from build123d import *

# Parameters (mm, degrees)
BOSS_EXTRUDE2_DEPTH = 8


with BuildPart() as part:
    # Sketch1 → Boss-Extrude2 (new body)
    with BuildSketch(Plane.XY):
        Polygon((0, 0), (-20, 0), (-20, 6), (-24, 6), (-24, 0), (-34.5, 0), (-34.5, 6), (-38.5, 6), (-38.5, -4), (0, -4), align=None)
    extrude(amount=BOSS_EXTRUDE2_DEPTH)

    # Mirror1: part across plane


with BuildPart() as part_1:
    add(part.part)
    add(part.part.mirror(Plane(origin=(0, 0, 0), x_dir=(0, 0, 1), z_dir=(1, 0, 0))))


solid = part_1.part
Could you check a few things on this model? Use its own coordinates, in mm. A direction names the side the tool comes from. Give positions to 0.01 mm unless a question says otherwise; leave off trailing zeros. Order: outer loops, then holes, each group sorted by start corner. A loop starts at its lowest first (then second) coordinate and runs counter-clockwise, first axis right, second up. Notation, with made-up numbers: (74.5, 14.5) -> (133.5, 14.5) arc R24 cw to (133.5, 37.5) -> close; hole circle Ø6 at (76.25, 36.5). An arc over 180 degrees is marked (long way). Answer in a Markdown table with one row per item. Add a question column.
Item 1: Imagine slicing it at A-A (y = 1). List the corners of the cut face in (x, z) for me.
Item 2: We'd pull the mould along X, two halves only. Please class faces 1 (the flat face through (38.5, 1, 4)), 2 (the flat face through (-24, 3, 4)), 3 (the flat face through (36, 6, 4)): pulls with the +X half, pulls with the -X half, needs draft (parallel to the pull), parting line crosses it, or undercut.
Item 3: For faces 4 (the flat face through (20, 3, 4)), 5 (the flat face through (1, -1, 0)), which set-ups out of +Z, -Z, +X, -X, +Y, -Y let a thin tool reach every point of the face, with its end or its side?
Item 4: Please list where these lines run through material, in increasing order: probe 1 along X at (y, z) = (3.25, 2.5); probe 2 along Y at (x, z) = (-19, 0.5).
Item 5: I'm going to push flat-ended pins straight in: P1, Ø3, axis at x = -30, z = 3, coming from the +Y side; P2, Ø2, axis at x = -30, y = 2, coming from the +Z side; P3, Ø4, axis at x = -25.5, y = 1, coming from the -Z side. Where does each tip first touch, or does it pass through?
Item 6: Imagine slicing it at B-B (z = 2.75). List the corners of the cut face in (x, y) for me.
Item 7: Imagine slicing it at C-C (x = -10). List the corners of the cut face in (y, z) for me.
Result:
| question | item | result |
|---|---|---|
| 1 | outline | (-38.5, 0) -> (-34.5, 0) -> (-34.5, 8) -> (-38.5, 8) -> close; (-24, 0) -> (-20, 0) -> (-20, 8) -> (-24, 8) -> close; (20, 0) -> (24, 0) -> (24, 8) -> (20, 8) -> close; (34.5, 0) -> (38.5, 0) -> (38.5, 8) -> (34.5, 8) -> close |
| 2 | face 1 | pulls with the +X half |
| 2 | face 2 | undercut |
| 2 | face 3 | needs draft |
| 3 | face 4 | +Z, -Z, +Y |
| 3 | face 5 | -Z, +X, -X, +Y, -Y |
| 4 | probe 1 | -38.5 to -34.5, -24 to -20, 20 to 24, 34.5 to 38.5 |
| 4 | probe 2 | -4 to 0 |
| 5 | P1 | y = 0 |
| 5 | P2 | through |
| 5 | P3 | z = 0 |
| 6 | outline | (-38.5, -4) -> (38.5, -4) -> (38.5, 6) -> (34.5, 6) -> (34.5, 0) -> (24, 0) -> (24, 6) -> (20, 6) -> (20, 0) -> (-20, 0) -> (-20, 6) -> (-24, 6) -> (-24, 0) -> (-34.5, 0) -> (-34.5, 6) -> (-38.5, 6) -> close |
| 7 | outline | (-4, 0) -> (0, 0) -> (0, 8) -> (-4, 8) -> close |
